Could you check a few things on this model? Use its own coordinates, in mm. Face numbers are marked on the shaded views. A direction names the side the tool comes from. Give positions to 0.01 mm unless a question says otherwise; leave off trailing zeros. Order: outer loops, then holes, each group sorted by start corner. A loop starts at its lowest first (then second) coordinate and runs counter-clockwise, first axis right, second up. Notation, with made-up numbers: (-33, 9.25) -> (-22, 9.25) arc R18 cw to (-22, 15.25) -> close; hole circle Ø10 at (15.5, 38). An arc over 180 degrees is marked (long way). One line per item, written item: value.
```python
from build123d import *

# Parameters (mm, degrees)
BOSS_EXTRU_1_DEPTH      = 9
ESQUISSE3_R             = 5
BOSS_EXTRU_3_DEPTH      = 8
ENL_V_MAT_EXTRU_1_DEPTH = 27.507114611
ENL_V_MAT_EXTRU_2_DEPTH = 2
BOSS_EXTRU_4_DEPTH      = 2
CHANFREIN1_SIZE         = 2


with BuildPart() as part:
    # Esquisse1 → Boss.-Extru.1 (new body)
    with BuildSketch(Plane(origin=(0, 0, 0), x_dir=(0, 1, 0), z_dir=(0, 0, 1))):
        with BuildLine():
            Line((-7.89, -10.855), (-7.89, 10.855))
            ThreePointArc((-7.89, 10.855), (0, 18.745), (7.89, 10.855))
            Line((7.89, 10.855), (7.89, -10.855))
            ThreePointArc((7.89, -10.855), (0, -18.745), (-7.89, -10.855))
        make_face()
    extrude(amount=BOSS_EXTRU_1_DEPTH)

    # Esquisse3 → Boss.-Extru.3 (add)
    with BuildSketch(Plane(origin=(0, 0, 0), x_dir=(1, 0, 0), z_dir=(0, 0, -1))):
        with Locations((10.855, 0)):
            Circle(ESQUISSE3_R)
    extrude(amount=BOSS_EXTRU_3_DEPTH)

    # Esquisse2 → Enlèv. mat.-Extru.1 (cut, through all)
    with BuildSketch(Plane.XY.offset(9)):
        Polygon((-10.855, 3.935), (-14.262809964, 1.9675), (-14.262809964, -1.9675), (-10.855, -3.935), (-7.447190036, -1.9675), (-7.447190036, 1.9675), align=None)
    extrude(amount=-ENL_V_MAT_EXTRU_1_DEPTH, mode=Mode.SUBTRACT)

    # Esquisse4 → Enlèv. mat.-Extru.2 (cut)
    with BuildSketch(Plane(origin=(0, 0, 0), x_dir=(1, 0, 0), z_dir=(0, 0, -1))):
        Polygon((-5.447190036, -3.122200538), (-5.447190036, 3.122200538), (-10.855, 6.244401077), (-16.262809964, 3.122200538), (-16.262809964, -3.122200538), (-10.855, -6.244401077), align=None)
    extrude(amount=-ENL_V_MAT_EXTRU_2_DEPTH, mode=Mode.SUBTRACT)

    # Esquisse5 → Boss.-Extru.4 (add)
    with BuildSketch(Plane.XY.offset(9)):
        with BuildLine():
            ThreePointArc((-10.855, -7.89), (-5.275927496, -5.579072504), (-2.965, 0))
            ThreePointArc((-2.965, 0), (-5.275927496, 5.579072504), (-10.855, 7.89))
            ThreePointArc((-10.855, 7.89), (-18.745, 0), (-10.855, -7.89))
        make_face()
        Polygon((-10.855, 3.935), (-7.447190036, 1.9675), (-7.447190036, -1.9675), (-10.855, -3.935), (-14.262809964, -1.9675), (-14.262809964, 1.9675), align=None, mode=Mode.SUBTRACT)
    extrude(amount=BOSS_EXTRU_4_DEPTH)

    # Chanfrein1
    chanfrein1_edges = [part.edges().sort_by_distance(p)[0] for p in [
        (-9.151095018, 2.95125, 11),
        (-7.447190036, 0, 11),
        (-9.151095018, -2.95125, 11),
        (-12.558904982, -2.95125, 11),
        (-14.262809964, 0, 11),
        (-12.558904982, 2.95125, 11),
    ]]
    chamfer(chanfrein1_edges, length=CHANFREIN1_SIZE - 0.0001)  # a hair under: the kernel refuses the full size


solid = part.part
```
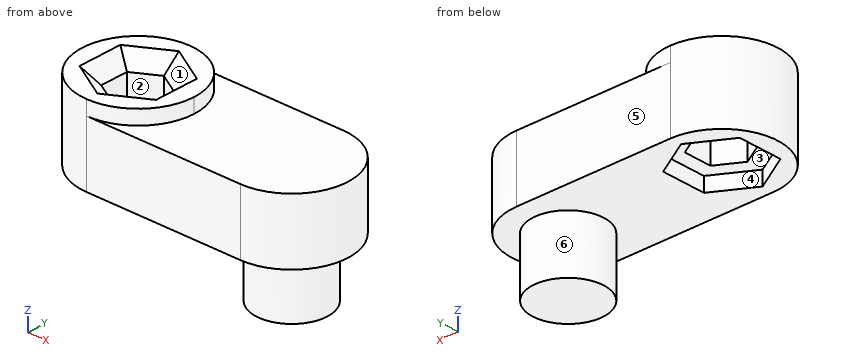
1) Suppose I cut it at B-B, the plane x = -8.5. Write out the boundary of the cut face in (y, z).
Answer below:
outline: (-7.89, 0) -> (-4.88, 0) -> (-4.88, 2) -> (-2.58, 2) -> (-2.58, 9) -> (-4.88, 11) -> (-7.53, 11) -> (-7.53, 9) -> (-7.89, 9) -> close; (2.58, 2) -> (4.88, 2) -> (4.88, 0) -> (7.89, 0) -> (7.89, 9) -> (7.53, 9) -> (7.53, 11) -> (4.88, 11) -> (2.58, 9) -> close
2) For the marked faces 1, 2 and 3, which set-ups out of +Z, -Z, +X, -X, +Y, -Y let a thin tool reach every point of the face, with its end or its side?
Answer below:
face 1: +Z
face 2: +Z, -Z
face 3: -Z
3) Suppose I cut it at C-C, the plane x = 6.5. Write out the boundary of the cut face in (y, z), then the cut area to 3 significant figures.
Answer below:
outline: (-7.89, 0) -> (-2.46, 0) -> (-2.46, -8) -> (2.46, -8) -> (2.46, 0) -> (7.89, 0) -> (7.89, 9) -> (-7.89, 9) -> close
area: 181 mm2
4) Suppose I cut it at A-A, the plane z = 5. Write out the boundary of the cut face in (x, y) (1 decimal), then the cut area to 3 significant figures.
Answer below:
outline: (-10.9, -7.9) -> (10.9, -7.9) arc R7.9 ccw to (10.9, 7.9) -> (-10.9, 7.9) arc R7.9 ccw to start; hole (-14.3, -2) -> (-10.9, -3.9) -> (-7.4, -2) -> (-7.4, 2) -> (-10.9, 3.9) -> (-14.3, 2) -> close
area: 498 mm2
5) For P1, Ø8.5, axis at x = -9, y = 1.5, coming from the -Z side; P2, Ø4, axis at x = -13, z = 7, coming from the +Y side; P3, Ø6, axis at y = 0.5, z = -4, coming from the +X side (3 decimals), each with a flat end and sliding along its axis, tell me the tip position at first contact or that it passes through.
Answer below:
P1: stops at z = 0
P2: stops at y = 7.89
P3: stops at x = 15.855
6) Suppose I cut it at D-D, the plane z = 9.5. Write out the boundary of the cut face in (x, y) (3 decimals), then the cut area to 3 significant figures.
Answer below:
outline: circle Ø15.78 at (-10.855, 0); hole (-14.763, -2.256) -> (-10.855, -4.512) -> (-6.947, -2.256) -> (-6.947, 2.256) -> (-10.855, 4.512) -> (-14.763, 2.256) -> close
area: 143 mm2
7) We'd pull the mould along X, two halves only. Please class the marked faces 4, 5 and 6: +X half, -X half, draft (parallel to the pull), parting line (faces both ways), or undercut.
Answer below:
face 4: undercut
face 5: draft
face 6: parting line
8) If I drill on line 1 along Z through (x, y) = (5.5, -7); line 2 along Y through (x, z) = (-11.5, 8.5); line 3 along Y through (x, z) = (-11, 8), over which ranges is the centre line in solid material (lowest first)?
Answer below:
line 1: z = 0 to 9
line 2: y = -7.86 to -3.56, 3.56 to 7.86
line 3: y = -7.89 to -3.85, 3.85 to 7.89
